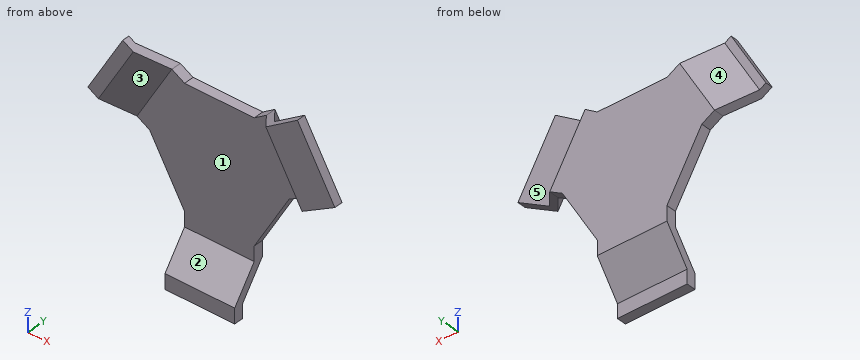
from build123d import *

# Parameters (mm, degrees)
BOSS_EXTRUDE1_DEPTH = 10
BOSS_EXTRUDE3_DEPTH = 69.34963783
BOSS_EXTRUDE4_DEPTH = 69.34963783
BOSS_EXTRUDE5_REACH = 181.774


with BuildPart() as part:
    # Sketch2 → Boss-Extrude1 (new body)
    with BuildSketch(Plane(origin=(0, 0, 0), x_dir=(1, 0, 0), z_dir=(0, 1, 0))):
        Polygon((-34.674818915, 60.058548104), (-34.674818915, 74.628755779), (34.674818915, 74.628755779), (34.674818915, 60.058548104), (69.34963783, 0), (81.964725461, -7.290440025), (46.802147984, -68.134366411), (34.674818915, -60.058548104), (-34.674818915, -60.058548104), (-47.2929889, -67.343651941), (-81.967807815, -7.285103837), (-69.34963783, 0), align=None)
    extrude(amount=BOSS_EXTRUDE1_DEPTH)

    # Sketch5 → Boss-Extrude3 (add)
    with BuildSketch(Plane(origin=(17.337409458, 0, 30.029274052), x_dir=(0.8660254037844373, 0, -0.5000000000000024), z_dir=(0.5000000000000024, 0, 0.8660254037844373))):
        Polygon((-74.628755779, 10), (-107.500686605, -9.402116298), (-114.804327341, -9.402116298), (-114.804327341, -16.610041857), (-102.770229552, -16.610041857), (-74.628755779, 0), align=None)
    extrude(amount=-BOSS_EXTRUDE3_DEPTH)

    # Sketch7 → Boss-Extrude4 (add)
    with BuildSketch(Plane.ZY.offset(34.674818915)):
        Polygon((-74.628755779, 10), (-106.637571533, -13.734668021), (-120.515633105, -13.734668021), (-120.515633105, -23.002237989), (-105.649808909, -23.002237989), (-74.628755779, 0), align=None)
    extrude(amount=-BOSS_EXTRUDE4_DEPTH)

    # Boss-Extrude5: up to this plane
    boss_extrude5_end = Plane(origin=(46.802147984, 10, 68.134366411), z_dir=(0.5542692655665835, 0, -0.8323374203099847))
    # Sketch8 → Boss-Extrude5 (add, up to the surface)
    with BuildSketch(Plane(origin=(17.362817345, 0, -30.043928978), x_dir=(-0.8658138519612032, 0, -0.500366239620644), z_dir=(0.500366239620644, 0, -0.8658138519612032)), mode=Mode.PRIVATE) as boss_extrude5_sk1:
        Polygon((-74.614084737, 10), (-103.818325668, -19.516175566), (-140.022146245, -19.516175566), (-140.022146245, -28.029543005), (-102.347404227, -28.029543005), (-74.614084737, 0), align=None)
    boss_extrude5_tool1 = split(extrude(boss_extrude5_sk1.sketch, amount=-BOSS_EXTRUDE5_REACH, mode=Mode.PRIVATE), bisect_by=boss_extrude5_end, keep=Keep.BOTH, mode=Mode.PRIVATE)
    add(boss_extrude5_tool1.solids().sort_by_distance((94.141781, -5.290236, 14.327735))[0])


solid = part.part
CAD build for the part. Positions are in the model's coordinates, mm. Face numbers are marked on the shaded views. A direction names the side the tool comes from. Coordinates: 2 decimals unless noted, no trailing zeros. Write each loop counter-clockwise with the first axis right and the second up, starting at its lowest first coordinate (ties: lowest second). Pieces come first, ordered by that corner, then holes. Notation, with made-up numbers: (50, 8.5) - (61, 8.5) arc R9 cw to (61, 21.5) - close; hole circle Ø11 at (22.5, -32). An arc over 180 degrees is marked (long way). Use a Markdown table: item, result. Add a question column.
Item 1: Band-saw the part on A-A, the plane y = -6.5. Give the cut face in (x, z) (3 decimals), and give its area (3 significant figures).
Item 2: Drill centre lines: L1, parallel to Y at x = -13.5, z = -1.5; L2, parallel to Y at x = 106.5, z = 80.5; L3, parallel to X at y = -15.5, z = 35.5. Where is each one in solid material? Low to high. Write a range as from..to.
Item 3: Band-saw the part on D-D, the plane z = 36. Give the cut face in (x, y), and give its area (3 significant figures).
Item 4: Flat gauge pins, fed straight in: pin 1 (8 mm diameter, centred on y = -2.5, z = 10, fed in from +X); pin 2 (4 mm diameter, centred on x = -16, z = -115, fed in from +Y); pin 3 (4 mm diameter, centred on x = 104.5, z = 62.5, fed in from +Y); pin 4 (2 mm diameter, centred on y = -2.5, z = -52.5, fed in from +X). Where does each tip first touch, or does it go through?
Item 5: Band-saw the part on C-C, the plane x = 4. Give the cut face in (y, z).
Item 6: Band-saw the part on B-B, the plane z = 71.5. Give the cut face in (x, y), and give its area (3 significant figures).
Item 7: Mould opens along X. For the marked faces 3, 4 and 5 say: pulls with the +X half, pulls with the -X half, needs draft (parallel to the pull), parting line crosses it, or undercut.
Item 8: 3-axis set-ups, long thin cutter, end or side, ignore diameter. For the marked faces 1 and 2: which of +Z, -Z, +X, -X, +Y, -Y reach the whole face in a straight line?
Numbers:
| question | item | result |
|---|---|---|
| 1 | outline | (-106.178, 21.263) - (-91.505, 12.791) - (-56.83, 72.85) - (-71.503, 81.321) - close; (-34.675, -96.881) - (34.675, -96.881) - (34.675, -83.395) - (-34.675, -83.395) - close; (52.166, 71.706) - (87.533, 10.508) - (96.1, 15.459) - (60.418, 77.201) - close |
| 1 | area | 2,810 mm2 |
| 2 | L1 | 0..10 |
| 2 | L2 | -28.03..-19.52 |
| 2 | L3 | -112.07..-96, 83.38..94.8 |
| 3 | outline | (-111.78, -16.61) - (-97.88, -16.61) - (-65.39, 0) - (65.37, 0) - (97.4, -28.03) - (131.64, -28.03) - (131.64, -19.52) - (99.1, -19.52) - (65.37, 10) - (-65.39, 10) - (-103.35, -9.4) - (-111.78, -9.4) - close |
| 3 | area | 2,350 mm2 |
| 4 | pin 1 | x = 93.41 |
| 4 | pin 2 | y = -13.73 |
| 4 | pin 3 | y = -19.52 |
| 4 | pin 4 | through |
| 5 | outline | (-23, -120.52) - (-13.73, -120.52) - (-13.73, -106.64) - (10, -74.63) - (10, 60.06) - (0, 60.06) - (0, -74.63) - (-23, -105.65) - close |
| 6 | outline | (-91.28, -16.61) - (-77.39, -16.61) - (-54.49, -4.91) - (-54.49, 5.09) - (-82.85, -9.4) - (-91.28, -9.4) - close; (51.86, -6.12) - (76.89, -28.03) - (120.4, -28.03) - (120.4, -19.52) - (78.59, -19.52) - (51.86, 3.88) - close |
| 6 | area | 959 mm2 |
| 7 | face 3 | undercut |
| 7 | face 4 | pulls with the -X half |
| 7 | face 5 | needs draft |
| 8 | face 1 | -Y |
| 8 | face 2 | +Z, +X, -X, -Y |
